```python
from build123d import *

# Parameters (mm, degrees)
F0_R     = 5
F0_R_2   = 3.175
F1_DEPTH = 5
F2_R     = 95
F2_R_2   = 92.5
F3_DEPTH = 38.23
F6_D     = 1.9939
F6_DEPTH = 13.58625
F6_TIP   = 0.5990279941
F7_D     = 12
F7_DEPTH = 13.59
F7_TIP   = 3.6051637142


with BuildPart() as f1:
    # F0 (on Top) → F1 (new body)
    with BuildSketch(Plane.XY):
        with BuildLine():
            ThreePointArc((54.7412050142, -77.6427747675), (84.3368676094, -43.7297697436), (95, 0))
            ThreePointArc((95, 0), (84.3368676094, 43.7297697436), (54.7412050142, 77.6427747675))
            ThreePointArc((54.7412050142, 77.6427747675), (0, 95), (-54.7412050142, 77.6427747675))
            ThreePointArc((-54.7412050142, 77.6427747675), (-95, 0), (-54.7412050142, -77.6427747675))
            ThreePointArc((-54.7412050142, -77.6427747675), (0, -95), (54.7412050142, -77.6427747675))
        make_face()
        Circle(F0_R, mode=Mode.SUBTRACT)
        with BuildLine():
            ThreePointArc((54.7412050142, 77.6427747675), (84.3368676094, 43.7297697436), (95, 0))
            ThreePointArc((95, 0), (84.3368676094, -43.7297697436), (54.7412050142, -77.6427747675))
            Line((54.7412050142, -77.6427747675), (137.3353012535, -19.4106936919))
            ThreePointArc((137.3353012535, -19.4106936919), (99.9, 0), (137.3353012535, 19.4106936919))
            Line((137.3353012535, 19.4106936919), (54.7412050142, 77.6427747675))
        make_face()
        with BuildLine():
            ThreePointArc((-54.7412050142, -77.6427747675), (-95, 0), (-54.7412050142, 77.6427747675))
            Line((-54.7412050142, 77.6427747675), (-137.3353012535, 19.4106936919))
            ThreePointArc((-137.3353012535, 19.4106936919), (-112.7175575641, 21.0842169024), (-99.9, 0))
            ThreePointArc((-99.9, 0), (-112.7175575641, -21.0842169024), (-137.3353012535, -19.4106936919))
            Line((-137.3353012535, -19.4106936919), (-54.7412050142, -77.6427747675))
        make_face()
        with BuildLine():
            ThreePointArc((147.4, 0), (144.7342169024, 10.9324424359), (137.3353012535, 19.4106936919))
            ThreePointArc((137.3353012535, 19.4106936919), (99.9, 0), (137.3353012535, -19.4106936919))
            ThreePointArc((137.3353012535, -19.4106936919), (144.7342169024, -10.9324424359), (147.4, 0))
        make_face()
        with Locations((123.65, 0)):
            Circle(F0_R_2, mode=Mode.SUBTRACT)
        with BuildLine():
            ThreePointArc((-99.9, 0), (-112.7175575641, 21.0842169024), (-137.3353012535, 19.4106936919))
            ThreePointArc((-137.3353012535, 19.4106936919), (-147.4, 0), (-137.3353012535, -19.4106936919))
            ThreePointArc((-137.3353012535, -19.4106936919), (-112.7175575641, -21.0842169024), (-99.9, 0))
        make_face()
        with Locations((-123.65, 0)):
            Circle(F0_R_2, mode=Mode.SUBTRACT)
    extrude(amount=F1_DEPTH)

    # F2 (on face) → F3 (join)
    with BuildSketch(Plane(origin=(0, 0, 0), x_dir=(1, 0, 0), z_dir=(0, 0, -1))):
        Circle(F2_R)
        Circle(F2_R_2, mode=Mode.SUBTRACT)
    extrude(amount=F3_DEPTH)

    # F6
    with Locations(Plane.XY.offset(5)):
        with Locations((-5.75, 5.75), (5.75, 5.75), (5.75, -5.75), (-5.75, -5.75)):
            Hole(F6_D / 2, depth=F6_DEPTH)
            with Locations((0, 0, -(F6_DEPTH + F6_TIP / 2))):  # 118° drill point
                Cone(0, F6_D / 2, F6_TIP, mode=Mode.SUBTRACT)

    # F7
    with Locations(Plane.XY.offset(5)):
        with Locations((-31.75, 0), (31.75, 0)):
            Hole(F7_D / 2, depth=F7_DEPTH)
            with Locations((0, 0, -(F7_DEPTH + F7_TIP / 2))):  # 118° drill point
                Cone(0, F7_D / 2, F7_TIP, mode=Mode.SUBTRACT)


solid = f1.part
```
For this review, take the finished solid that the model builds, in its own axes (mm). A direction names the side the tool comes from. Give positions to 0.01 mm unless a question says otherwise; leave off trailing zeros. Loops run counter-clockwise (first coordinate to the right, second up) from the corner with the lowest first, then second, coordinate; pieces in that order, holes last. Notation, with made-up numbers: M 11.25,49.25 L 30.25,49.25 A15 cw 30.25,64.25 Z; hole C -36,44 d4. An arc over 180 degrees is marked long. One line per item, written item: value. Start each with the question number.
Q1. Draft analysis for pull direction Y (two halves, no side actions). For faces 3 (the face through (126.68, 0.95, 2.46)), 4 (the face through (111, 6, 0)), 5 (the face through (95.46, -48.934, 2.465)), state which applies: released by +Y, released by -Y, zero draft, split by the parting line, or undercut.
Q2. Add section B-B (z = -14). Give the boundary of the cut face in (x, y).
Q3. Add section A-A (x = -31.75). Give the boundary of the cut face in (y, z).
Q4. Machinability: for faces 1 (the face through (96.616, 48.119, 2.465)), 2 (the face through (49.727, -77.996, -18.847)), which of the approach directions +Z, -Z, +X, -X, +Y, -Y give a long, thin tool a straight path to every point of the face, cutting with its end or side? Answer none if there is none.
Q5. Add section D-D (y = 36). Give the boundary of the cut face in (x, z), and give its area (3 significant figures).
Q6. Add section C-C (x = -123.65). Give the boundary of the cut face in (y, z) (3 decimals), and give its area (3 significant figures).
Q7. Clearance check with flat-ended pins moving along their axes: pin 1 Ø16 at (x, y) = (0, 0) entering from -Z; pin 2 Ø1 at (x, z) = (21, 0.5) entering from +Y; pin 3 Ø4 at (x, z) = (-80.5, -25) entering from +Y. State where each tip first meets the part, or that it passes through.
Q8. For L1, parallel to Y at x = -5.75, z = 1.8; L2, parallel to Y at x = 0, z = 3.3; L3, parallel to X at y = -2, z = -35, list the stretches that pass through material, from the lowest coordinate up.
Reply:
1. face 3: undercut
1. face 4: zero draft
1. face 5: released by -Y
2. outline: C 0,0 d190; hole C 0,0 d185
3. outline: M -89.54,-38.23 L -86.88,-38.23 L -86.88,0 L -6,0 L -6,5 L -89.54,5 Z; M 6,0 L 86.88,0 L 86.88,-38.23 L 89.54,-38.23 L 89.54,5 L 6,5 Z
4. face 1: +Z, -Z, +X, +Y
4. face 2: -Z
5. outline: M -113.81,0 L -87.91,0 L -87.91,-38.23 L -85.21,-38.23 L -85.21,0 L 85.21,0 L 85.21,-38.23 L 87.91,-38.23 L 87.91,0 L 113.81,0 L 113.81,5 L -113.81,5 Z
5. area: 1,350 mm²
6. outline: M -29.059,0 L -3.175,0 L -3.175,5 L -29.059,5 Z; M 3.175,0 L 29.059,0 L 29.059,5 L 3.175,5 Z
6. area: 259 mm²
7. pin 1: z = 0
7. pin 2: y = 92.76
7. pin 3: y = 53.5
8. L1: -94.83 to -6.75, -4.75 to 4.75, 6.75 to 94.83
8. L2: -95 to -5, 5 to 95
8. L3: -94.98 to -92.48, 92.48 to 94.98
